Can you work these out from the model? Positions are in its coordinate system, mm. A direction names the side the tool comes from. Give positions to 0.01 mm unless a question says otherwise; leave off trailing zeros. Loops run counter-clockwise (first coordinate to the right, second up) from the corner with the lowest first, then second, coordinate; pieces in that order, holes last. Notation, with made-up numbers: M 4,-10 L 36,-10 A17 ccw 36,9 Z; hole C 0,-21 d11. An arc over 180 degrees is marked long. Put each result on its own line as item: value. Start each with the question number.
1) For P1, Ø0.6, axis at x = -74.5, z = 48, coming from the -Y side; P2, Ø15, axis at x = 28.5, y = 34.5, coming from the +Z side; P3, Ø12, axis at x = -30, y = 46, coming from the -Z side, each with a flat end and sliding along its axis, tell me the tip position at first contact or that it passes through.
2) For faces 4 (the cylindrical face through (122.719, 26.143, -47.594)), 5 (the flat face through (123, 27, 1)), 6 (the cylindrical face through (-72.451, -1.232, 52.846)), which set-ups out of +Z, -Z, +X, -X, +Y, -Y let a thin tool reach every point of the face, with its end or its side?
3) Imagine slicing it at C-C (x = -55). Write out the boundary of the cut face in (y, z).
4) Imagine slicing it at A-A (z = 21). Write out the boundary of the cut face in (x, y), then the cut area to 3 significant figures.
5) If we mould it in two halves opening along Z, with no side actions, what happens to faces 1 (the flat face through (125, 26, 1)), 2 (the cylindrical face through (79.549, -1.232, -49.154)), 3 (the cylindrical face through (-122.719, 26.143, 47.594))? For each: +Z half, -Z half, draft (parallel to the pull), parting line (faces both ways), or undercut.
6) Imagine slicing it at B-B (y = 44.5). Write out the boundary of the cut face in (x, z), then the cut area to 3 significant figures.
7) Imagine slicing it at D-D (x = -20). Write out the boundary of the cut face in (y, z).
8) Please list where these lines run through material, in increasing order: line 1 along X through (y, z) = (-1.7, -51); line 2 along Z through (x, y) = (68.5, 44.5); line 3 along Z through (x, y) = (-76, -1.85). Write a range as from..to.
from build123d import *

# Parameters (mm, degrees)
BOSS_EXTRUDE1_DEPTH     = 52
FILLET1_R               = 1
SHELL1_T                = -2
SKETCH2_R               = 9
SKETCH2_R_2             = 4
BOSS_EXTRUDE2_DEPTH     = 2.5
SKETCH3_R               = 14.5
CUT_EXTRUDE1_DEPTH      = 175.439101121
CUT_EXTRUDE2_DEPTH      = 149.084435374
CUT_EXTRUDE2_DEPTH_BACK = 149.084435374
SKETCH4_R               = 14.5


with BuildPart() as part:
    # Sketch1 → Boss-Extrude1 (new body)
    with BuildSketch(Plane(origin=(0, 0, 0), x_dir=(1, 0, 0), z_dir=(0, 1, 0))):
        with BuildLine():
            Line((125, -42), (125, 42))
            ThreePointArc((125, 42), (122.656854249, 47.656854249), (117, 50))
            Line((117, 50), (-117, 50))
            ThreePointArc((-117, 50), (-122.656854249, 47.656854249), (-125, 42))
            Line((-125, 42), (-125, -42))
            ThreePointArc((-125, -42), (-122.656854249, -47.656854249), (-117, -50))
            Line((-117, -50), (117, -50))
            ThreePointArc((117, -50), (122.656854249, -47.656854249), (125, -42))
        make_face()
    extrude(amount=BOSS_EXTRUDE1_DEPTH)

    # Fillet1
    fillet1_edges = [part.edges().sort_by_distance(p)[0] for p in [
        (0, 0, -50),
        (122.656854249, 0, -47.656854249),
        (125, 0, 0),
        (122.656854249, 0, 47.656854249),
        (0, 0, 50),
        (-122.656854249, 0, 47.656854249),
        (-125, 0, 0),
        (-122.656854249, 0, -47.656854249),
    ]]
    fillet(fillet1_edges, radius=FILLET1_R)

    # Shell1
    shell1_openings = [part.faces().sort_by_distance(p)[0] for p in [
        (0, 52, 0),
    ]]
    offset(amount=SHELL1_T, openings=shell1_openings, kind=Kind.INTERSECTION)

    # Sketch2 → Boss-Extrude2 (add)
    # profile 1 of 4: a face of its own
    with BuildSketch(Plane.XZ):
        with Locations(Location((76, 51, 0), (0, 0, 192.839588407))):
            Circle(SKETCH2_R)
        with Locations(Location((76, 51, 0), (0, 0, 330))):
            Circle(SKETCH2_R_2, mode=Mode.SUBTRACT)
    # profile 2 of 4: a face of its own
    with BuildSketch(Plane.XZ):
        with Locations(Location((76, -51, 0), (0, 0, 90))):
            Circle(SKETCH2_R)
        with Locations(Location((76, -51, 0), (0, 0, 90))):
            Circle(SKETCH2_R_2, mode=Mode.SUBTRACT)
    # profile 3 of 4: a face of its own
    with BuildSketch(Plane.XZ):
        with Locations(Location((-76, -51, 0), (0, 0, 167.160411593))):
            Circle(SKETCH2_R)
        with Locations(Location((-76, -51, 0), (0, 0, 30))):
            Circle(SKETCH2_R_2, mode=Mode.SUBTRACT)
    # profile 4 of 4: a face of its own
    with BuildSketch(Plane.XZ):
        with Locations(Location((-76, 51, 0), (0, 0, 90))):
            Circle(SKETCH2_R)
        with Locations(Location((-76, 51, 0), (0, 0, 90))):
            Circle(SKETCH2_R_2, mode=Mode.SUBTRACT)
    extrude(amount=BOSS_EXTRUDE2_DEPTH)

    # Sketch3 → Cut-Extrude1 (cut, through all)
    with BuildSketch(Plane(origin=(0, 0, -50), x_dir=(-1, 0, 0), z_dir=(0, 0, -1))):
        with Locations((-55, 25.3)):
            Circle(SKETCH3_R)
        with Locations((0, 25.3)):
            Circle(SKETCH3_R)
        with Locations((55, 25.3)):
            Circle(SKETCH3_R)
    extrude(amount=-CUT_EXTRUDE1_DEPTH, mode=Mode.SUBTRACT)

    # Sketch4 → Cut-Extrude2 (cut, two sides: drawn at the far end of the back side and taken through both)
    with BuildSketch(Plane(origin=(0, 0, 0), x_dir=(0, 0, -1), z_dir=(1, 0, 0)).offset(-CUT_EXTRUDE2_DEPTH_BACK)):
        with Locations(Location((31, 25.3, 0), (0, 0, 40.657248638))):
            Circle(SKETCH4_R)
        with Locations(Location((-31, 25.3, 0), (0, 0, 139.342751362))):
            Circle(SKETCH4_R)
    extrude(amount=CUT_EXTRUDE2_DEPTH + CUT_EXTRUDE2_DEPTH_BACK, mode=Mode.SUBTRACT)


solid = part.part
Recorded:
1. P1: y = 0
1. P2: z = 50
1. P3: z = -50
2. face 4: -Z, +X, +Y, -Y
2. face 5: +Y
2. face 6: -Y
3. outline: M 0,-49 A1 ccw 1,-50 L 10.8,-50 L 10.8,-48 L 2,-48 L 2,48 L 10.8,48 L 10.8,50 L 1,50 A1 ccw 0,49 Z; M 39.8,-50 L 52,-50 L 52,-48 L 39.8,-48 Z; M 39.8,48 L 52,48 L 52,50 L 39.8,50 Z
4. outline: M -125,1 A1 ccw -124,0 L 124,0 A1 ccw 125,1 L 125,14.8 L 123,14.8 L 123,2 L -123,2 L -123,14.8 L -125,14.8 Z; M -125,35.8 L -123,35.8 L -123,52 L -125,52 Z; M 123,35.8 L 125,35.8 L 125,52 L 123,52 Z
4. area: 616 mm²
5. face 1: draft
5. face 2: undercut
5. face 3: +Z half
6. outline: M -125,-42 A8 ccw -117,-50 L 117,-50 A8 ccw 125,-42 L 125,42 A8 ccw 117,50 L -117,50 A8 ccw -125,42 Z; hole M -123,-42 A6 ccw -117,-48 L 117,-48 A6 ccw 123,-42 L 123,42 A6 ccw 117,48 L -117,48 A6 ccw -123,42 Z
6. area: 1,360 mm²
7. outline: M 0,-49 A1 ccw 1,-50 L 52,-50 L 52,-48 L 2,-48 L 2,48 L 52,48 L 52,50 L 1,50 A1 ccw 0,49 Z
8. line 1: -85..-80, -72..-67, 67..72, 80..85
8. line 2: -50..-48, 48..50
8. line 3: -60..-55, -47..-42, 42..47, 55..60
